Read the model definition and answer for the solid it produces. Units are mm, in the model's axes. Coordinates: 2 decimals unless noted, no trailing zeros. Order: outer loops, then holes, each group sorted by start corner. A loop starts at its lowest first (then second) coordinate and runs counter-clockwise, first axis right, second up. Notation, with made-up numbers: (5.5, 2) -> (50.5, 2) arc R11 ccw to (50.5, 15) -> close; hole circle Ø4 at (11.5, 35). An arc over 180 degrees is marked (long way). Answer in a Markdown table with one row per item.
from build123d import *

# Parameters (mm, degrees)
F1_DEPTH = 58.42


with BuildPart() as f1:
    # F0 (on Top) → F1 (new body)
    with BuildSketch(Plane.XY):
        with BuildLine():
            Line((-20.150693, -5.465834), (32.733693, -5.465834))
            ThreePointArc((32.733693, -5.465834), (33.051588, -2.74113), (33.157765, 0))
            ThreePointArc((33.157765, 0), (27.878729, 18.608382), (13.614477, 31.672504))
            Line((13.614477, 31.672504), (-18.171751, 31.672504))
            ThreePointArc((-18.171751, 31.672504), (-19.169745, 31.15171), (-20.150693, 30.59948))
            Line((-20.150693, 30.59948), (-20.150693, -5.465834))
        make_face()
    extrude(amount=-F1_DEPTH)


solid = f1.part
Q1. Consider line 1 (X direction, y = 5.5, z = -52.5); line 2 (X direction, y = 27.5, z = -31); line 3 (Y direction, x = 16, z = -56). Determine where each line is inside the solid, lowest interval first.
Outcome:
| item | result |
|---|---|
| line 1 | -20.15 to 32.73 |
| line 2 | -20.15 to 20.07 |
| line 3 | -5.47 to 30.36 |
Q2. The part is cut by section A-A (z = -22). Write down the section's boundary in (x, y), then the cut area to 3 significant figures.
Outcome:
| item | result |
|---|---|
| outline | (-20.15, -5.47) -> (32.73, -5.47) arc R35.44 ccw to (33.16, 0) arc R35.44 ccw to (13.61, 31.67) -> (-18.17, 31.67) arc R35.44 ccw to (-20.15, 30.6) -> close |
| area | 1,800 mm² |
Q3. The part is cut by section C-C (x = 23.5). Write down the section's boundary in (y, z).
Outcome:
| item | result |
|---|---|
| outline | (-5.47, -58.42) -> (24.31, -58.42) -> (24.31, 0) -> (-5.47, 0) -> close |
Q4. The part is cut by section B-B (y = 27.5). Write down the section's boundary in (x, z).
Outcome:
| item | result |
|---|---|
| outline | (-20.15, -58.42) -> (20.07, -58.42) -> (20.07, 0) -> (-20.15, 0) -> close |
